Part model, mm, in its own coordinate system. A direction names the side the tool comes from. Round coordinates to 2 decimals unless told otherwise and drop trailing zeros. Write each loop counter-clockwise with the first axis right and the second up, starting at its lowest first coordinate (ties: lowest second). Pieces come first, ordered by that corner, then holes. Notation, with made-up numbers: (8, 73.25) -> (40, 73.25) arc R13 cw to (40, 78.25) -> close; hole circle Ø4 at (-15, 23). An arc over 180 degrees is marked (long way). Return JSON: item names as keys, results as strings. Group by question number.
(1) Drop flat-ended pins along their axis: pin 1 Ø4 at (x, y) = (35, 2.5) entering from -Z; pin 2 Ø4 at (x, y) = (-80, 16) entering from +Z; pin 3 Ø5 at (x, y) = (-71.5, 16.5) entering from -Z. Give the stop position or say it passes through.
(2) Mould opens along Z. For faces 1 (the flat face through (80, -20, 40)), 2 (the flat face through (95, 1, 1)), 3 (the flat face through (-90, -30, 32)) say: +Z half, -Z half, draft (parallel to the pull), parting line (faces both ways), or undercut.
(3) Saw through at B-B (x = -79). List the corners of the cut face in (y, z).
(4) Saw through at D-D (x = 48.5). List the corners of the cut face in (y, z), plus the area to 3 significant figures.
(5) Saw through at C-C (z = 5.5). List the corners of the cut face in (x, y), plus the area to 3 significant figures.
(6) Saw through at A-A (y = -17.5). List the corners of the cut face in (x, z), plus the area to 3 significant figures.
(7) Drill centre lines: L1, parallel to X at y = 11.5, z = 32; L2, parallel to Y at x = -48.5, z = 0; L3, parallel to Y at x = -67, z = 34. Where is each one in solid material? Low to high. Write a range as from..to.
(8) Tool access for faces 4 (the flat face through (-70, -30, -32)), 5 (the cylindrical face through (1.4, 36.95, 15.32)), 6 (the flat face through (90, -30, 32)): list every direction of +Z, -Z, +X, -X, +Y, -Y with a clear straight run to the whole face (end or side of a thin tool).
from build123d import *

# Parameters (mm, degrees)
IZIM1_W                     = 200
IZIM1_H                     = 40
IZIM2_R                     = 38
KES_EKSTR_ZYON2_DEPTH       = 190
IZIM3_W                     = 30
IZIM3_H                     = 20
KES_EKSTR_ZYON3_DEPTH       = 10
Y_KSEKLIK_EKSTR_ZYON1_DEPTH = 10
AYNALAMA2_COPY_1_DEPTH      = 10


with BuildPart() as part:
    # Çizim1 → Döndür1 (revolve)
    with BuildSketch(Plane.XY):
        with Locations((0, 20)):
            Rectangle(IZIM1_W, IZIM1_H)
    revolve(axis=Axis((100, 0, 0), (-1, 0, 0)))

    # Çizim2 → Kes-Ekstrüzyon2 (cut)
    with BuildSketch(Plane(origin=(-95, 0, 0), x_dir=(0, 0, -1), z_dir=(1, 0, 0))):
        Circle(IZIM2_R)
    extrude(amount=KES_EKSTR_ZYON2_DEPTH, mode=Mode.SUBTRACT)

    # Çizim3 → Kes-Ekstrüzyon3 (cut)
    with BuildSketch(Plane(origin=(0, 40, 0), x_dir=(1, 0, 0), z_dir=(0, 1, 0))):
        with Locations((-75, 0)):
            Rectangle(IZIM3_W, IZIM3_H)
    extrude(amount=-KES_EKSTR_ZYON3_DEPTH, mode=Mode.SUBTRACT)

    # Çizim5 → Yükseklik-Ekstrüzyon1 (add, symmetric)
    with BuildSketch(Plane(origin=(80, 0, 0), x_dir=(0, 0, -1), z_dir=(1, 0, 0))):
        with BuildLine():
            ThreePointArc((0, -40), (-28.284271247, -28.284271247), (-40, 0))
            Line((-40, 0), (-40, -40))
            Line((-40, -40), (0, -40))
        make_face()
    y_kseklik_ekstr_zyon1 = extrude(amount=Y_KSEKLIK_EKSTR_ZYON1_DEPTH, both=True)

    # Aynalama1: Yükseklik-Ekstrüzyon1 across plane
    add(y_kseklik_ekstr_zyon1.mirror(Plane.XY))

    # Aynalama2: Yükseklik-Ekstrüzyon1 across plane
    add(y_kseklik_ekstr_zyon1.mirror(Plane(origin=(0, 0, 0), x_dir=(0, 0, 1), z_dir=(1, 0, 0))))

    # Aynalama2 copy 1 sketch → Aynalama2 copy 1 (add, symmetric)
    with BuildSketch(Plane.ZY.offset(80)):
        with BuildLine():
            ThreePointArc((0, -40), (-28.284271247, -28.284271247), (-40, 0))
            Line((-40, 0), (-40, -40))
            Line((-40, -40), (0, -40))
        make_face()
    extrude(amount=AYNALAMA2_COPY_1_DEPTH, both=True)


solid = part.part
Computed values:
{
 "1": {"pin 1": "z = -40", "pin 2": "z = 37.47", "pin 3": "z = -37.47"},
 "2": {"face 1": "+Z half", "face 2": "undercut", "face 3": "draft"},
 "3": {"outline": "(-40, -40) -> (0, -40) arc R40 ccw to (38.73, -10) -> (36.66, -10) arc R38 cw (long way) to (36.66, 10) -> (38.73, 10) arc R40 ccw to (0, 40) -> (-40, 40) -> close"},
 "4": {"outline": "circle Ø80 at (0, 0); hole circle Ø76 at (0, 0)", "area": "490 mm2"},
 "5": {"outline": "(-100, -39.62) -> (-90, -39.62) -> (-90, -40) -> (-70, -40) -> (-70, -39.62) -> (70, -39.62) -> (70, -40) -> (90, -40) -> (90, -39.62) -> (100, -39.62) -> (100, 39.62) -> (-60, 39.62) -> (-60, 37.6) -> (95, 37.6) -> (95, -37.6) -> (-95, -37.6) -> (-95, 37.6) -> (-90, 37.6) -> (-90, 39.62) -> (-100, 39.62) -> close", "area": "1,510 mm2"},
 "6": {"outline": "(-100, -35.97) -> (-90, -35.97) -> (-90, -40) -> (-70, -40) -> (-70, -35.97) -> (70, -35.97) -> (70, -40) -> (90, -40) -> (90, -35.97) -> (100, -35.97) -> (100, 35.97) -> (90, 35.97) -> (90, 40) -> (70, 40) -> (70, 35.97) -> (-70, 35.97) -> (-70, 40) -> (-90, 40) -> (-90, 35.97) -> (-100, 35.97) -> close; hole (-95, -33.73) -> (95, -33.73) -> (95, 33.73) -> (-95, 33.73) -> close", "area": "1,890 mm2"},
 "7": {"L1": "-100..-95, 95..100", "L2": "-40..-38, 38..40", "L3": "-21.07..-16.97, 16.97..21.07"},
 "8": {"face 4": "-Z, -Y", "face 5": "none", "face 6": "+Z, +X, -Y"}
}
